Part model, mm, in its own coordinate system. A direction names the side the tool comes from. Give positions to 0.01 mm unless a question says otherwise; leave off trailing zeros. Order: outer loops, then holes, each group sorted by start corner. A loop starts at its lowest first (then second) coordinate and runs counter-clockwise, first axis right, second up. Notation, with made-up numbers: (81.5, -36.75) - (102.5, -36.75) arc R24 cw to (102.5, 2.25) - close; hole circle Ø1 at (80, -26.5). An arc over 180 degrees is marked (long way). Use one line per item in the form item = value. Start each with the question number.
1. Band-saw the part on A-A, the plane y = 23. List the corners of the cut face in (x, z).
2. Drill centre lines: line 1 (Z direction, x = 0, y = -76.5); line 2 (X direction, y = -73.8, z = 0); line 3 (X direction, y = 43.5, z = 2.25). Where is each one in solid material? Low to high.
3. Pin check, flat tip, straight feed: P1, Ø4, axis at x = -0.5, y = 55.5, coming from the +Z side. Stop position of the tip, or through.
4. Tool access for faces 1 (the face through (0.748, 75.325, -0.976)), 2 (the face through (-3.5, 1, 0)), 3 (the face through (-0.748, -75.325, -0.976)): list every direction of +Z, -Z, +X, -X, +Y, -Y with a clear straight run to the whole face (end or side of a thin tool).
Autodesk Inventor part; units mm, degrees
ref_plane "YZ Plane" through (0, 0, 0) normal (1, 0, 0) x (0, 1, 0)
ref_plane "XZ Plane" through (0, 0, 0) normal (0, 1, 0) x (-1, 0, 0)
ref_plane "XY Plane" through (0, 0, 0) normal (0, 0, 1) x (1, 0, 0)
sketch "スケッチ1" plane through (0, 0, 0) normal (1, 0, 0) x (0, 1, 0)
  line L0 (-78.5, 0) -> (78.5, 0)
  line L1 (0, 0) -> (0, 4.0415) construction
  line L2 (-78.1874, 4.0415) -> (-78.5, 3.5)
  line L3 (-78.5, 3.5) -> (-78.5, 0)
  line L4 (-78.1874, 4.0415) -> (78.1874, 4.0415)
  line L5 (78.1874, 4.0415) -> (78.5, 3.5)
  line L6 (78.5, 3.5) -> (78.5, 0)
  dimension "d1" = 3.5
  dimension "d2" = 4.0415
  dimension "d3" = 30
  dimension "d4" = 157
revolve "回転1" add sketch "スケッチ1" angle 360 about axis through (0, -78.5, 0) along (0, 1, 0)
sketch "スケッチ2" plane through (0, 78.5, 0) normal (0, 1, 0) x (1, 0, 0)
  circle A0 centre (0, 0) radius 4.0415
  line L0 (0, -4.0415) -> (-3.5, -2.0207)
  line L1 (-3.5, -2.0207) -> (-3.5, 2.0207)
  line L2 (-3.5, 2.0207) -> (0, 4.0415)
  line L3 (0, 4.0415) -> (3.5, 2.0207)
  line L4 (3.5, 2.0207) -> (3.5, -2.0207)
  line L5 (3.5, -2.0207) -> (0, -4.0415)
  point P0 (0, 0)
  point P1 (0, 0)
  point P2 (3.5, -2.0207)
  point P3 (3.5, 2.0207)
  point P4 (3.5, 2.0207)
  point P5 (0, 4.0415)
  point P6 (0, 4.0415)
  point P7 (-3.5, 2.0207)
  point P8 (-3.5, 2.0207)
  point P9 (-3.5, -2.0207)
  point P10 (-3.5, -2.0207)
  point P11 (0, 0)
extrude "押し出し1" cut sketch "スケッチ2" against normal through all contours A0 L4 | L3 A0 | A0 L5 | L2 A0 | A0 L0 | L1 A0
hole "穴1" at (0, 78.5, 0) direction (0, -1, 0) diameter 2.459 depth 6 tip angle 118 countersink diameter 3 countersink angle 90
mirror "ミラー1" about plane through (0, 0, 0) normal (0, 1, 0) of "穴1"
equation "\"d2\" = 1.1547 * d1"
properties part number "SLSBF7-157-M3-N3" material "ステンレス鋼 AISI 304"
From the geometry:
q1.outline = (-3.5, -2.02) - (0, -4.04) - (3.5, -2.02) - (3.5, 2.02) - (0, 4.04) - (-3.5, 2.02) - close
q2.line_1 = -4.04 to -1.23, 1.23 to 4.04
q2.line_2 = -3.5 to -1.23, 1.23 to 3.5
q2.line_3 = -3.1 to 3.1
q3.P1 = 4.04
q4.face_1 = +Y
q4.face_2 = +Z, -Z, -X, +Y, -Y
q4.face_3 = -Y
